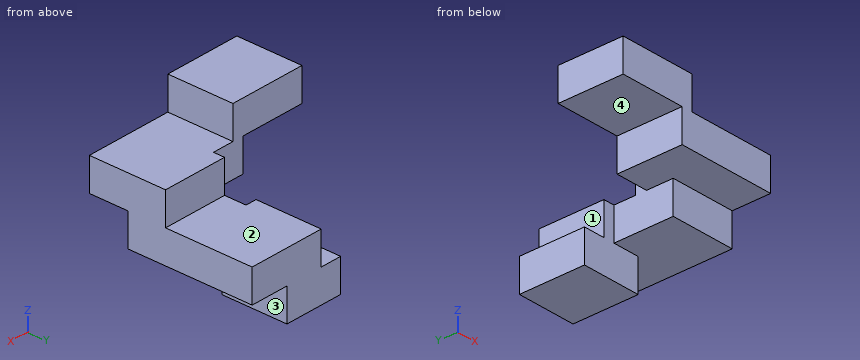
Autodesk Inventor part; units mm, degrees
ref_plane "YZ Plane" through (0, 0, 0) normal (1, 0, 0) x (0, 1, 0)
ref_plane "XZ Plane" through (0, 0, 0) normal (0, 1, 0) x (-1, 0, 0)
ref_plane "XY Plane" through (0, 0, 0) normal (0, 0, 1) x (1, 0, 0)
sketch "草圖15" plane through (0, 0, 0) normal (0, 0, 1) x (1, 0, 0)
  line L0 (5, -5) -> (-5, -5)
  line L1 (-5, -5) -> (-5, 5)
  line L2 (-5, 5) -> (5, 5)
  line L3 (5, 5) -> (5, -5)
  line L4 (5, -5) -> (-5, 5) construction
  line L5 (-5, -5) -> (5, 5) construction
  line L6 (25, -25) -> (-25, -25)
  line L7 (-25, -25) -> (-25, 25)
  line L8 (-25, 25) -> (25, 25)
  line L9 (25, 25) -> (25, -25)
  line L10 (25, -25) -> (-25, 25) construction
  line L11 (-25, -25) -> (25, 25) construction
  line L12 (-25, -25) -> (-1.6, -25)
  line L13 (-1.6, -25) -> (-1.6, -5)
  line L14 (-1.6, -5) -> (-25, -5)
  line L15 (-25, -5) -> (-25, -25)
  line L16 (25, -25) -> (-1.6, -25)
  line L17 (-1.6, -5) -> (25, -5)
  line L18 (25, -5) -> (25, -25)
  line L19 (25, -25) -> (5, -25)
  line L20 (5, -25) -> (5, -1.6)
  line L21 (5, -1.6) -> (25, -1.6)
  line L22 (25, -1.6) -> (25, -25)
  line L23 (25, 25) -> (5, 25)
  line L24 (5, 25) -> (5, -1.6)
  line L25 (25, -1.6) -> (25, 25)
  line L26 (25, 25) -> (1.6, 25)
  line L27 (1.6, 25) -> (1.6, 5)
  line L28 (1.6, 5) -> (25, 5)
  line L29 (25, 5) -> (25, 25)
  line L30 (-25, 25) -> (1.6, 25)
  line L31 (1.6, 5) -> (-25, 5)
  line L32 (-25, 5) -> (-25, 25)
  line L33 (-5, -5) -> (-25, -5)
  line L34 (-25, -5) -> (-25, -25)
  line L35 (-25, -25) -> (-5, -25)
  line L36 (-5, -25) -> (-5, -5)
  line L37 (-1.6, -25) -> (-13.2, -25)
  line L38 (-13.2, -25) -> (-13.2, -5)
  line L39 (-13.2, -5) -> (-1.6, -5)
  line L40 (-1.6, -5) -> (-1.6, -25)
  line L41 (5, -1.6) -> (25, -1.6)
  line L42 (25, -1.6) -> (25, -13.2)
  line L43 (25, -13.2) -> (5, -13.2)
  line L44 (5, -13.2) -> (5, -1.6)
  line L45 (1.6, 5) -> (13.2, 5)
  line L46 (13.2, 5) -> (13.2, 25)
  line L47 (13.2, 25) -> (1.6, 25)
  line L48 (1.6, 25) -> (1.6, 5)
  line L49 (1.6, 5) -> (-5, 5)
  line L50 (-5, 5) -> (-5, 25)
  line L51 (-5, 25) -> (1.6, 25)
  line L52 (1.6, 25) -> (1.6, 5)
  point P0 (0, 0)
  point P1 (0, 0)
  point P2 (-1.6, -25)
  point P3 (-25, 5)
  point P4 (-5, 5)
  point P5 (-5, -25)
  point P6 (5, 5)
  point P7 (-5, -25)
  point P8 (-13.2, -25)
  point P9 (25, -13.2)
  point P10 (-5, 25)
  point P11 (-5, 5)
  point P12 (5, 5)
  point P13 (13.2, 5)
  point P14 (13.2, 25)
  dimension "d38" = 10
  dimension "d39" = 20
  dimension "d40" = 1.6
  dimension "d42" = 1.6
  dimension "d48" = 1.6
  dimension "d54" = 0
  dimension "d55" = 11.6
  dimension "d56" = 11.6
  dimension "d57" = 11.6
  dimension "d58" = 10
extrude "擠出10" add sketch "草圖15" against normal blind 10 contours L13 L6 L36 L0 | L36 L6 L38 L14 | L38 L6 L7 L14
extrude "擠出11" add sketch "草圖15" against normal blind 10 from surface at -10 contours L20 L6 L13 L0 | L3 L21 L9 L17 | L17 L9 L43 L20 | L13 L6 L36 L0 | L43 L9 L6 L20
extrude "擠出12" add sketch "草圖15" against normal blind 10 from surface at -20 contours L3 L21 L9 L17 | L17 L9 L43 L20 | L3 L28 L9 L21 | L2 L27 L8 L24 | L24 L8 L46 L28 | L46 L8 L9 L28
extrude "擠出13" add sketch "草圖15" against normal blind 10 from surface at -30 contours L2 L27 L8 L24 | L24 L8 L46 L28 | L50 L8 L27 L2
equation "\"d39\" = width"
equation "\"d55\" = stack"
equation "\"d56\" = stack"
equation "\"d57\" = stack"
equation "\"d44\" = height"
equation "\"d46\" = height"
equation "\"d50\" = height"
equation "\"d52\" = height"
equation "\"width\" = 20"
equation "\"height\" = 10"
equation "\"gap\" = 1.6"
equation "\"stack\" = 11.6"
properties part number "Template_ladder_2"
Input: part model. Units: mm. Frame: model coordinates. Face numbers are marked on the shaded views. A direction names the side the tool comes from. Give positions to 0.01 mm unless a question says otherwise; leave off trailing zeros. Order: outer loops, then holes, each group sorted by start corner. A loop starts at its lowest first (then second) coordinate and runs counter-clockwise, first axis right, second up.
1. Line query: probe 1 along X at (y, z) = (14, -21); probe 2 along Y at (x, z) = (-1, -16); probe 3 along Z at (x, y) = (17, -4). Output: solid intervals per line, ascending.
Computed:
probe 1: x = 1.6 to 25
probe 2: y = -25 to -5
probe 3: z = -30 to -10
2. Cut plane A-A (x = 18.5). Return loops of the section in (y, z).
Computed:
outline: (-25, -20) - (-13.2, -20) - (-13.2, -30) - (25, -30) - (25, -20) - (-1.6, -20) - (-1.6, -10) - (-25, -10) - close
3. Pin query (flat end, axial travel): pin 1 Ø6 at (x, y) = (-11, -10.5) entering from -Z; pin 2 Ø5.5 at (y, z) = (-3.5, -23.5) entering from -X; pin 3 Ø5 at (y, z) = (-14, -15.5) entering from -X. Return the tip coordinate at first contact, or that it passes through.
Computed:
pin 1: stops at z = -10
pin 2: stops at x = 5
pin 3: stops at x = -5
4. Set-up query: the marked faces 1, 2, 3 and 4. Return all of +Z, -Z, +X, -X, +Y, -Y with unobstructed straight access to the full face (end or side cutting, diameter ignored); none if empty.
Computed:
face 1: +Z, -X, +Y, -Y
face 2: +Z, +X, -X, +Y
face 3: -Z, +X, +Y, -Y
face 4: -Z, -X, +Y, -Y
5. Cut plane C-C (z = -17). Return loops of the section in (x, y).
Computed:
outline: (-5, -25) - (25, -25) - (25, -1.6) - (5, -1.6) - (5, -5) - (-5, -5) - close
6. Cut plane D-D (x = 10.5). Return loops of the section in (y, z), and give its area (3 significant figures).
Computed:
outline: (-25, -20) - (-13.2, -20) - (-13.2, -30) - (5, -30) - (5, -40) - (25, -40) - (25, -20) - (-1.6, -20) - (-1.6, -10) - (-25, -10) - close
area: 816 mm2
7. Cut plane B-B (y = -17). Return loops of the section in (x, z), and give its area (3 significant figures).
Computed:
outline: (-25, -10) - (-5, -10) - (-5, -20) - (25, -20) - (25, -10) - (-1.6, -10) - (-1.6, 0) - (-25, 0) - close
area: 534 mm2
